The model under review builds one solid part; all positions refer to its coordinate system, in mm. A direction names the side the tool comes from. Coordinates: 2 decimals unless noted, no trailing zeros. Order: outer loops, then holes, each group sorted by start corner. A loop starts at its lowest first (then second) coordinate and runs counter-clockwise, first axis right, second up. Notation, with made-up numbers: M 0,62.25 L 13,62.25 A25 cw 13,95.25 Z; hole C 22,78.25 d8. An arc over 180 degrees is marked long. Answer as CSV lines item,"result". Start each with the question number.
Q1. Consider section D-D on z = 10. Write out the cut boundary in (x, y), and give its area (3 significant figures).
Q2. The part is to be moulded in two halves that separate along Z. For faces 5 (the face through (18, 33.5, 0)), 6 (the face through (17.514, 29.099, 17.454)), 7 (the face through (7.81, 19.72, -1.73)), say which applies: +Z half, -Z half, draft (parallel to the pull), parting line (faces both ways), or undercut.
Q3. Wall thickness on L1, parallel to Z at x = 0, y = 26.5; L2, parallel to X at y = 25, z = 0; L3, parallel to X at y = 16.5, z = 0: over which ranges is each line inside the solid? List them lowest first. Write a range as [from, to].
Q4. Consider section B-B on x = 0. Write out the cut boundary in (y, z).
Q5. Consider section A-A on z = 0. Write out the cut boundary in (x, y), and give its area (3 significant figures).
Q6. Consider section C-C on y = 29. Write out the cut boundary in (x, z).
Q7. Machinability: for faces 1 (the face through (-17.486, 29.099, 17.454)), 2 (the face through (-8, 18, 10)), 3 (the face through (18, 24.5, 0)), 4 (the face through (-17, 33.5, 0)), which of the approach directions +Z, -Z, +X, -X, +Y, -Y give a long, thin tool a straight path to every point of the face, cutting with its end or side? Answer none if there is none.
Q8. For P1, Ø4, axis at y = 16.5, z = 18, coming from the +X side; P2, Ø12, axis at y = 11, z = -13.5, coming from the +X side; P3, Ø1, axis at x = -17.5, z = 2, coming from the -Y side, all flat-tipped, find the tip position at first contact; note any pin that passes through.
from build123d import *

# Parameters (mm, degrees)
ESBO_O1_R                = 12.5
RESSALTO_EXTRUS_O1_DEPTH = 30
ESBO_O2_R                = 8
CORTE_EXTRUS_O1_DEPTH    = 15
ESBO_O3_W                = 3
ESBO_O3_H                = 5
CORTE_EXTRUS_O2_DEPTH    = 6.5
ESBO_O4_R                = 8
CORTE_EXTRUS_O3_DEPTH    = 35.820970693
ESBO_O5_W                = 25
ESBO_O5_H                = 25
RESSALTO_EXTRUS_O2_DEPTH = 12
ESBO_O6_W                = 25
ESBO_O6_H                = 25
RESSALTO_EXTRUS_O3_DEPTH = 10
ESBO_O7_R                = 8
CORTE_EXTRUS_O4_DEPTH    = 29.222331583
ESBO_O8_W                = 45
ESBO_O8_H                = 22
RESSALTO_EXTRUS_O4_DEPTH = 25
ESBO_O9_W                = 45.089311088
ESBO_O9_H                = 22
RESSALTO_EXTRUS_O5_DEPTH = 4
ESBO_O10_W               = 45.089311088
ESBO_O10_H               = 22
RESSALTO_EXTRUS_O6_DEPTH = 4
ESBO_O11_W               = 33
ESBO_O11_H               = 45
RESSALTO_EXTRUS_O7_DEPTH = 22
ESBO_O12_W               = 4
ESBO_O12_H               = 0.089311088
CORTE_EXTRUS_O5_DEPTH    = 49.790485687
RESSALTO_EXTRUS_O8_DEPTH = 2
RESSALTO_EXTRUS_O9_START = 2
RESSALTO_EXTRUS_O9_DEPTH = 2
ESBO_O15_R               = 8
CORTE_EXTRUS_O6_DEPTH    = 37.530966229


with BuildPart() as part:
    # Esboço1 → Ressalto-extrusão1 (new body)
    with BuildSketch(Plane(origin=(0, 0, 0), x_dir=(1, 0, 0), z_dir=(0, 1, 0))):
        with Locations(Location((0, 0, 0), (0, 0, 270))):
            Circle(ESBO_O1_R)
    extrude(amount=RESSALTO_EXTRUS_O1_DEPTH)

    # Esboço2 → Corte-extrusão1 (cut)
    with BuildSketch(Plane(origin=(0, 30, 0), x_dir=(1, 0, 0), z_dir=(0, 1, 0))):
        with Locations(Location((0, 0, 0), (0, 0, 270))):
            Circle(ESBO_O2_R)
    extrude(amount=-CORTE_EXTRUS_O1_DEPTH, mode=Mode.SUBTRACT)

    # Esboço3 → Corte-extrusão2 (cut)
    with BuildSketch(Plane.XZ):
        Rectangle(ESBO_O3_W, ESBO_O3_H)
    extrude(amount=-CORTE_EXTRUS_O2_DEPTH, mode=Mode.SUBTRACT)

    # Esboço4 → Corte-extrusão3 (cut, through all)
    with BuildSketch(Plane(origin=(0, 30, 0), x_dir=(1, 0, 0), z_dir=(0, 1, 0))):
        with Locations(Location((0, 0, 0), (0, 0, 270))):
            Circle(ESBO_O4_R)
    extrude(amount=-CORTE_EXTRUS_O3_DEPTH, mode=Mode.SUBTRACT)

    # Esboço5 → Ressalto-extrusão2 (add)
    with BuildSketch(Plane(origin=(0, 30, 0), x_dir=(1, 0, 0), z_dir=(0, 1, 0))):
        Rectangle(ESBO_O5_W, ESBO_O5_H)
    extrude(amount=-RESSALTO_EXTRUS_O2_DEPTH)

    # Esboço6 → Ressalto-extrusão3 (add)
    with BuildSketch(Plane(origin=(0, 30, 0), x_dir=(1, 0, 0), z_dir=(0, 1, 0))):
        Rectangle(ESBO_O6_W, ESBO_O6_H)
    extrude(amount=RESSALTO_EXTRUS_O3_DEPTH)

    # Esboço7 → Corte-extrusão4 (cut, through all)
    with BuildSketch(Plane.XZ.offset(-18)):
        with Locations(Location((0, 0, 0), (0, 0, 90))):
            Circle(ESBO_O7_R)
    extrude(amount=-CORTE_EXTRUS_O4_DEPTH, mode=Mode.SUBTRACT)

    # Esboço8 → Ressalto-extrusão4 (add)
    with BuildSketch(Plane(origin=(12.5, 0, 0), x_dir=(0, 0, -1), z_dir=(1, 0, 0))):
        with Locations((0.044655544, 29)):
            Rectangle(ESBO_O8_W, ESBO_O8_H)
    extrude(amount=-RESSALTO_EXTRUS_O4_DEPTH)

    # Esboço9 → Ressalto-extrusão5 (add)
    with BuildSketch(Plane.ZY.offset(12.5)):
        with Locations((0, 29)):
            Rectangle(ESBO_O9_W, ESBO_O9_H)
    extrude(amount=RESSALTO_EXTRUS_O5_DEPTH)

    # Esboço10 → Ressalto-extrusão6 (add)
    with BuildSketch(Plane(origin=(12.5, 0, 0), x_dir=(0, 0, -1), z_dir=(1, 0, 0))):
        with Locations((0, 29)):
            Rectangle(ESBO_O10_W, ESBO_O10_H)
    extrude(amount=RESSALTO_EXTRUS_O6_DEPTH)

    # Esboço11 → Ressalto-extrusão7 (add)
    with BuildSketch(Plane(origin=(0, 40, 0), x_dir=(1, 0, 0), z_dir=(0, 1, 0))):
        with Locations((0, 0.044655544)):
            Rectangle(ESBO_O11_W, ESBO_O11_H)
    extrude(amount=-RESSALTO_EXTRUS_O7_DEPTH)

    # Esboço12 → Corte-extrusão5 (cut, through all)
    with BuildSketch(Plane(origin=(0, 40, 0), x_dir=(1, 0, 0), z_dir=(0, 1, 0))):
        with Locations((-14.5, -22.5)):
            Rectangle(ESBO_O12_W, ESBO_O12_H)
        with Locations((14.5, -22.5)):
            Rectangle(ESBO_O12_W, ESBO_O12_H)
    extrude(amount=-CORTE_EXTRUS_O5_DEPTH, mode=Mode.SUBTRACT)

    # Esboço13 → Ressalto-extrusão8 (add)
    with BuildSketch(Plane.ZY.offset(16.5)):
        with BuildLine():
            Line((-13.044655544, 33.5), (12.955344456, 33.5))
            ThreePointArc((12.955344456, 33.5), (17.455344456, 29), (12.955344456, 24.5))
            Line((12.955344456, 24.5), (-13.044655544, 24.5))
            ThreePointArc((-13.044655544, 24.5), (-17.544655544, 29), (-13.044655544, 33.5))
        make_face()
    extrude(amount=RESSALTO_EXTRUS_O8_DEPTH)

    # Esboço14 → Ressalto-extrusão9 (add)
    with BuildSketch(Plane(origin=(16.5, 0, 0), x_dir=(0, 0, -1), z_dir=(1, 0, 0)).offset(RESSALTO_EXTRUS_O9_START)):
        with BuildLine():
            Line((-12.955344456, 24.5), (13.044655544, 24.5))
            ThreePointArc((13.044655544, 24.5), (17.544655544, 29), (13.044655544, 33.5))
            Line((13.044655544, 33.5), (-12.955344456, 33.5))
            ThreePointArc((-12.955344456, 33.5), (-17.455344456, 29), (-12.955344456, 24.5))
        make_face()
    extrude(amount=-RESSALTO_EXTRUS_O9_DEPTH)

    # Esboço15 → Corte-extrusão6 (cut, through all)
    with BuildSketch(Plane.XZ.offset(-18)):
        with Locations(Location((0, 0, 0), (0, 0, 90))):
            Circle(ESBO_O15_R)
    extrude(amount=-CORTE_EXTRUS_O6_DEPTH, mode=Mode.SUBTRACT)


solid = part.part
Evaluation:
1,outline,"M -18.5,24.5 L -16.5,24.5 L -16.5,18 L -7.5,18 L -7.5,0 L 7.5,0 L 7.5,18 L 16.5,18 L 16.5,24.5 L 18.5,24.5 L 18.5,33.5 L 16.5,33.5 L 16.5,40 L -16.5,40 L -16.5,33.5 L -18.5,33.5 Z"
1,area,"1,030 mm²"
2,face 5,"draft"
2,face 6,"+Z half"
2,face 7,"undercut"
3,L1,"z = [-22.54, -8], [8, 22.46]"
3,L2,"x = [-18.5, -8], [8, 18.5]"
3,L3,"x = [-12.5, -8], [8, 12.5]"
4,outline,"M 0,-12.5 L 18,-12.5 L 18,-22.54 L 40,-22.54 L 40,-8 L 0,-8 Z; M 0,8 L 40,8 L 40,22.46 L 18,22.46 L 18,12.5 L 0,12.5 Z"
5,outline,"M -18.5,24.5 L -16.5,24.5 L -16.5,18 L -12.5,18 L -12.5,0 L -8,0 L -8,40 L -16.5,40 L -16.5,33.5 L -18.5,33.5 Z; M 8,0 L 12.5,0 L 12.5,18 L 16.5,18 L 16.5,24.5 L 18.5,24.5 L 18.5,33.5 L 16.5,33.5 L 16.5,40 L 8,40 Z"
5,area,"572 mm²"
6,outline,"M -18.5,-17.54 L -16.5,-17.54 L -16.5,-22.54 L 16.5,-22.54 L 16.5,-17.54 L 18.5,-17.54 L 18.5,17.46 L 16.5,17.46 L 16.5,22.46 L -16.5,22.46 L -16.5,17.46 L -18.5,17.46 Z; hole C 0,0 d16"
7,face 1,"+Z, -X"
7,face 2,"-Y"
7,face 3,"+Z, -Z, +X, -Y"
7,face 4,"+Z, -Z, -X, +Y"
8,P1,"stops at x = 16.5"
8,P2,"stops at x = 10"
8,P3,"stops at y = 24.5"
